Source: CAD feature listing. Evaluate the final solid. Frame: model axes, mm. Give positions to 0.01 mm unless a question says otherwise; leave off trailing zeros. Write each loop counter-clockwise with the first axis right and the second up, starting at its lowest first coordinate (ties: lowest second). Pieces come first, ordered by that corner, then holes. Notation, with made-up numbers: (-2, 25.5) - (54, 25.5) arc R24 cw to (54, 50.5) - close; hole circle Ø2 at (70, 53). An arc over 180 degrees is marked (long way). One line per question, with ' | ' between items. Start each with the question number.
(1) Section A-A, the plane x = 112. Return loops of the section in (y, z) (3 decimals), plus the area to 3 significant figures.
(2) Section B-B, the plane z = -30. Return loops of the section in (x, y) (3 decimals).
(3) Section C-C, the plane x = 453. Return loops of the section in (y, z) (3 decimals).
(4) Ray query, line 1 (Z direction, x = 307, y = 12) (3 decimals); line 2 (Y direction, x = 234, z = -30) (3 decimals); line 3 (X direction, y = 14.25, z = -40). Return the intervals inside material, ascending. Write a range as [from, to].
(5) Pin query (flat end, axial travel): pin 1 (1 mm diameter, centred on x = 293, z = -20, fed in from +Y) (3 decimals); pin 2 (4 mm diameter, centred on x = 440.8, y = 21.23, fed in from +Z); pin 3 (1.6 mm diameter, centred on x = 475.5, z = -1.5, fed in from +Y). Return the tip coordinate at first contact, or that it passes through.
Autodesk Inventor part; units mm, degrees
ref_plane "YZ Plane" through (0, 0, 0) normal (1, 0, 0) x (0, 1, 0)
ref_plane "XZ Plane" through (0, 0, 0) normal (0, 1, 0) x (-1, 0, 0)
ref_plane "XY Plane" through (0, 0, 0) normal (0, 0, 1) x (1, 0, 0)
sketch "Sketch1" plane through (0, 0, 0) normal (1, 0, 0) x (0, 1, 0)
  line L0 (0, 0) -> (25.4, 0)
  line L1 (25.4, 0) -> (25.4, -42.799)
  line L2 (25.4, -42.799) -> (0, -42.799)
  line L3 (0, -42.799) -> (0, 0)
  line L4 (25.4, -3.175) -> (3.175, -3.175)
  line L5 (3.175, -3.175) -> (3.175, -39.624)
  line L6 (3.175, -39.624) -> (25.4, -39.624)
  line L7 (25.4, -39.624) -> (25.4, -3.175)
  dimension "d0" = 25.4
  dimension "d1" = 42.799
  dimension "d2" = 22.225
  dimension "d3" = 36.449
  dimension "d4" = 3.175
extrude "Extrusion1" add sketch "Sketch1" along normal blind 495.3 contours L0 L1 L4 L5 L6 L2 L3
sketch "Sketch2" plane through (0, 0, 0) normal (0, 0, 1) x (1, 0, 0)
  line L0 (0, 25.4) -> (0, 0)
  line L1 (0, 0) -> (495.3, 0)
  line L2 (495.3, 25.4) -> (495.3, 0)
  line L3 (0, 25.4) -> (495.3, 25.4)
  line L4 (486.41, 25.4) -> (444.5, 25.4)
  line L5 (444.5, 25.4) -> (444.5, 6.35)
  line L6 (444.5, 6.35) -> (486.41, 6.35)
  line L7 (486.41, 6.35) -> (486.41, 25.4)
  circle A0 centre (490.2962, 21.2344) radius 2.413
  circle A1 centre (490.2962, 11.2344) radius 2.413
  circle A2 centre (440.7962, 21.2344) radius 2.413
  circle A3 centre (440.7962, 11.2344) radius 2.413
  dimension "d7" = 8.89
  dimension "d8" = 25.4
  dimension "d9" = 19.05
  dimension "d10" = 50.8
  dimension "d11" = 4.826
  dimension "d12" = 4.826
  dimension "d13" = 4.1656
  dimension "d14" = 10
  dimension "d15" = 4.826
  dimension "d16" = 4.826
  dimension "d26" = 5.0038
  dimension "d27" = 5.0038
  dimension "d28" = 49.5
  dimension "d29" = 49.5
  dimension "d30" = 10
extrude "Extrusion2" cut sketch "Sketch2" against normal blind 12.7 contours L3 L7 L6 L5 | A0 | A1 | A2 | A3
sketch "Sketch3" plane through (0, 0, -42.799) normal (0, 0, -1) x (-1, 0, 0)
  line L0 (0, 0) -> (0, 25.4)
  line L1 (0, 25.4) -> (-495.3, 25.4)
  line L2 (-495.3, 0) -> (-495.3, 25.4)
  line L3 (0, 0) -> (-495.3, 0)
  circle A0 centre (-475.5896, 16.2306) radius 3.175
  point P0 (0, 0)
  dimension "d21" = 6.35
  dimension "d22" = 19.7104
  dimension "d23" = 9.1694
extrude "Extrusion3" cut sketch "Sketch3" against normal blind 12.7 contours A0
equation "\"d12\" = d11"
equation "\"d15\" = d11"
equation "\"d16\" = d11"
equation "\"d27\" = d26"
equation "\"d29\" = d28"
equation "\"d30\" = d14"
properties part number "ArmProto1.2"
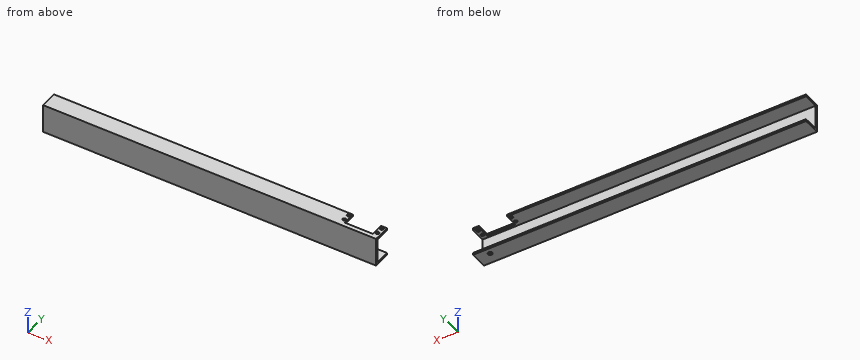
Check sheet entries:
1) outline: (0, -42.799) - (25.4, -42.799) - (25.4, -39.624) - (3.175, -39.624) - (3.175, -3.175) - (25.4, -3.175) - (25.4, 0) - (0, 0) - close | area: 277 mm²
2) outline: (0, 0) - (495.3, 0) - (495.3, 3.175) - (0, 3.175) - close
3) outline: (0, -42.799) - (25.4, -42.799) - (25.4, -39.624) - (3.175, -39.624) - (3.175, -3.175) - (6.35, -3.175) - (6.35, 0) - (0, 0) - close
4) line 1: [-42.799, -39.624], [-3.175, 0] | line 2: [0, 3.175] | line 3: [0, 473.11], [478.07, 495.3]
5) pin 1: y = 3.175 | pin 2: z = -39.62 | pin 3: y = 6.35
